Read the model definition and answer for the solid it produces. Units are mm, in the model's axes. Give positions to 0.01 mm unless a question says otherwise; leave off trailing zeros. Order: outer loops, then holes, each group sorted by start corner. A loop starts at its lowest first (then second) coordinate and runs counter-clockwise, first axis right, second up. Notation, with made-up numbers: (78.5, 33.5) -> (120.5, 33.5) arc R21 ccw to (120.5, 46.5) -> close; hole circle Ø3 at (80.5, 24.25). An arc over 180 degrees is marked (long way). One line per item, written item: value. Start each with the question number.
from build123d import *

# Parameters (mm, degrees)
SKETCH1_W           = 40
SKETCH1_H           = 4
BOSS_EXTRUDE1_DEPTH = 9
CUT_EXTRUDE1_REACH  = 43.195
SKETCH2_R           = 3


with BuildPart() as part:
    # Sketch1 → Boss-Extrude1 (new body)
    with BuildSketch(Plane(origin=(0, 0, 0), x_dir=(1, 0, 0), z_dir=(0, 1, 0))):
        with Locations((20, 2)):
            Rectangle(SKETCH1_W, SKETCH1_H)
    extrude(amount=BOSS_EXTRUDE1_DEPTH)

    # Sketch2 → Cut-Extrude1 (cut, up to next)
    with BuildSketch(Plane(origin=(0, 0, -4), x_dir=(-1, 0, 0), z_dir=(0, 0, -1)), mode=Mode.PRIVATE) as cut_extrude1_sk1:
        with Locations((-20, 4.5)):
            Circle(SKETCH2_R)
    cut_extrude1_tool1 = extrude(cut_extrude1_sk1.sketch, amount=-CUT_EXTRUDE1_REACH, mode=Mode.PRIVATE) & part.part
    add(cut_extrude1_tool1.solids().sort_by_distance((20, 4.5, -4))[0], mode=Mode.SUBTRACT)


solid = part.part
Item 1: Find section A-A on x = 20. Write down the section's boundary in (y, z), then the cut area to 3 significant figures.
Item 2: Find the intervals of material crossed by line 1 (Y direction, x = 20, z = -2.9); line 2 (X direction, y = 1.75, z = -1.85); line 3 (X direction, y = 5.75, z = -1.45), in increasing order. Write a range as from..to.
Item 3: For a pull along Y with two mould halves and no side action, classify faces 1 (the cylindrical face through (22.4, 2.7, -2)), 2 (the flat face through (20, 9, -2)), 3 (the flat face through (0, 4, -2)), 4 (the flat face through (20, 0, -2)) as +Y half, -Y half, draft (parallel to the pull), parting line (faces both ways), or undercut.
Item 4: Find section B-B on y = 4.5. Write down the section's boundary in (x, z), then the cut area to 3 significant figures.
Item 5: Find section C-C on z = -2.6. Write down the section's boundary in (x, y), then the cut area to 3 significant figures.
Checks:
1. outline: (0, -4) -> (1.5, -4) -> (1.5, 0) -> (0, 0) -> close; (7.5, -4) -> (9, -4) -> (9, 0) -> (7.5, 0) -> close
1. area: 12.0 mm2
2. line 1: 0..1.5, 7.5..9
2. line 2: 0..18.8, 21.2..40
2. line 3: 0..17.27, 22.73..40
3. face 1: undercut
3. face 2: +Y half
3. face 3: draft
3. face 4: -Y half
4. outline: (0, -4) -> (17, -4) -> (17, 0) -> (0, 0) -> close; (23, -4) -> (40, -4) -> (40, 0) -> (23, 0) -> close
4. area: 136 mm2
5. outline: (0, 0) -> (40, 0) -> (40, 9) -> (0, 9) -> close; hole circle Ø6 at (20, 4.5)
5. area: 332 mm2
